from build123d import *

# Parameters (mm, degrees)
BOSS_EXTRUDE1_DEPTH = 3.175


with BuildPart() as part:
    # Sketch1 → Boss-Extrude1 (new body)
    with BuildSketch(Plane.XY):
        Polygon((-203.3016, -8.62965), (-228.7016, -8.62965), (-228.7016, -46.135925), (222.1484, -46.135925), (222.1484, -52.409725), (-228.7016, -52.409725), (-228.7016, -63.32855), (228.7016, -63.32855), (228.7016, -8.62965), (203.3016, -8.62965), (203.3016, -5.65785), (228.7016, -5.65785), (228.7016, 5.65785), (203.3016, 5.65785), (203.3016, 8.62965), (228.7016, 8.62965), (228.7016, 63.32855), (-228.7016, 63.32855), (-228.7016, 52.409725), (222.1484, 52.409725), (222.1484, 46.135925), (-228.7016, 46.135925), (-228.7016, 8.62965), (-203.3016, 8.62965), (-203.3016, 5.65785), (-228.7016, 5.65785), (-228.7016, -5.65785), (-203.3016, -5.65785), align=None)
        Polygon((222.1484, -39.582725), (222.1484, -15.9766), (196.7484, -15.9766), (196.7484, 15.9766), (222.1484, 15.9766), (222.1484, 39.582725), (-222.1484, 39.582725), (-222.1484, 15.9766), (-196.7484, 15.9766), (-196.7484, -15.9766), (-222.1484, -15.9766), (-222.1484, -39.582725), align=None, mode=Mode.SUBTRACT)
    extrude(amount=BOSS_EXTRUDE1_DEPTH)


solid = part.part
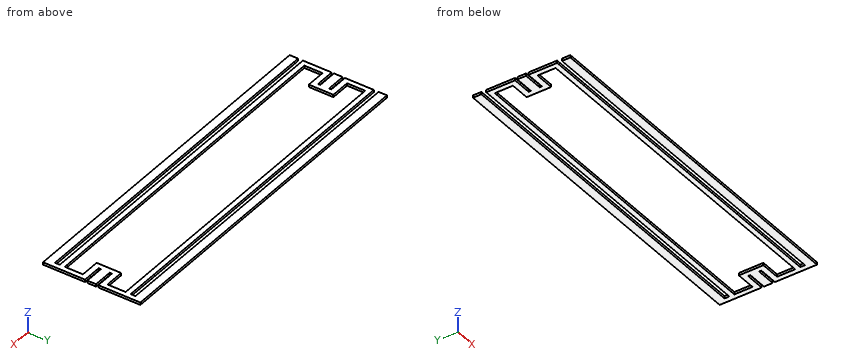
Work out the finished part from the listing and answer in its coordinate system (mm). Round coordinates to 2 decimals unless told otherwise and drop trailing zeros. Order: outer loops, then holes, each group sorted by start corner. A loop starts at its lowest first (then second) coordinate and runs counter-clockwise, first axis right, second up. Notation, with made-up numbers: M 81.25,-31.5 L 100.25,-31.5 A33 ccw 100.25,1.5 Z; hole C 73.25,16 d3. An arc over 180 degrees is marked long. Put each result on its own line as item: value. Start each with the question number.
Q1. Straight lines are drawn through the part: L1, parallel to Y at x = -169.5, z = 1.1; L2, parallel to Y at x = -200, z = 0.2; L3, parallel to X at y = -26, z = 0.3. For each, find the intervals that lie inside material, in ascending order. Write a range as [from, to].
Q2. Flat-ended cylindrical pins translate along their axes: pin 1 (1.5 mm diameter, centred on y = 7, z = 1, fed in from -X); pin 2 (0.9 mm diameter, centred on y = -6.5, z = 2, fed in from +X); pin 3 (1.6 mm diameter, centred on y = -48, z = 2, fed in from -X). Find the tip coordinate at first contact, or state that the pin passes through.
Q3. Section B-B, the plane y = 34.5 is taken. Write down the section's boundary in (x, z) (3 decimals).
Q4. Section A-A, the plane x = -17.5 is taken. Write down the section's boundary in (y, z) (3 decimals).
Findings below:
1. L1: y = [-63.33, -52.41], [-46.14, -39.58], [39.58, 46.14], [52.41, 63.33]
1. L2: y = [-63.33, -52.41], [-46.14, -39.58], [-15.98, 15.98], [39.58, 46.14], [52.41, 63.33]
1. L3: x = [-228.7, -222.15], [222.15, 228.7]
2. pin 1: stops at x = -203.3
2. pin 2: stops at x = 203.3
2. pin 3: stops at x = 222.15
3. outline: M -228.702,0 L -222.148,0 L -222.148,3.175 L -228.702,3.175 Z; M 222.148,0 L 228.702,0 L 228.702,3.175 L 222.148,3.175 Z
4. outline: M -63.329,0 L -52.41,0 L -52.41,3.175 L -63.329,3.175 Z; M -46.136,0 L -39.583,0 L -39.583,3.175 L -46.136,3.175 Z; M 39.583,0 L 46.136,0 L 46.136,3.175 L 39.583,3.175 Z; M 52.41,0 L 63.329,0 L 63.329,3.175 L 52.41,3.175 Z
